Geometry: see drawing. Coordinates: mm, zero at the bounding-box minimum. Coordinates: 2 decimals unless noted, no trailing zeros. Order: outer loops, then holes, each group sorted by start corner. A loop starts at its lowest first (then second) coordinate and runs counter-clockwise, first axis right, second up. Notation, with made-up numbers: (-12.5, 81) -> (13.5, 81) arc R20 cw to (13.5, 110) -> close; hole circle Ø7 at (4, 47). An arc over 180 degrees is marked (long way). Write each question's results on one line, items separated by ' | '. Start each with the question number.
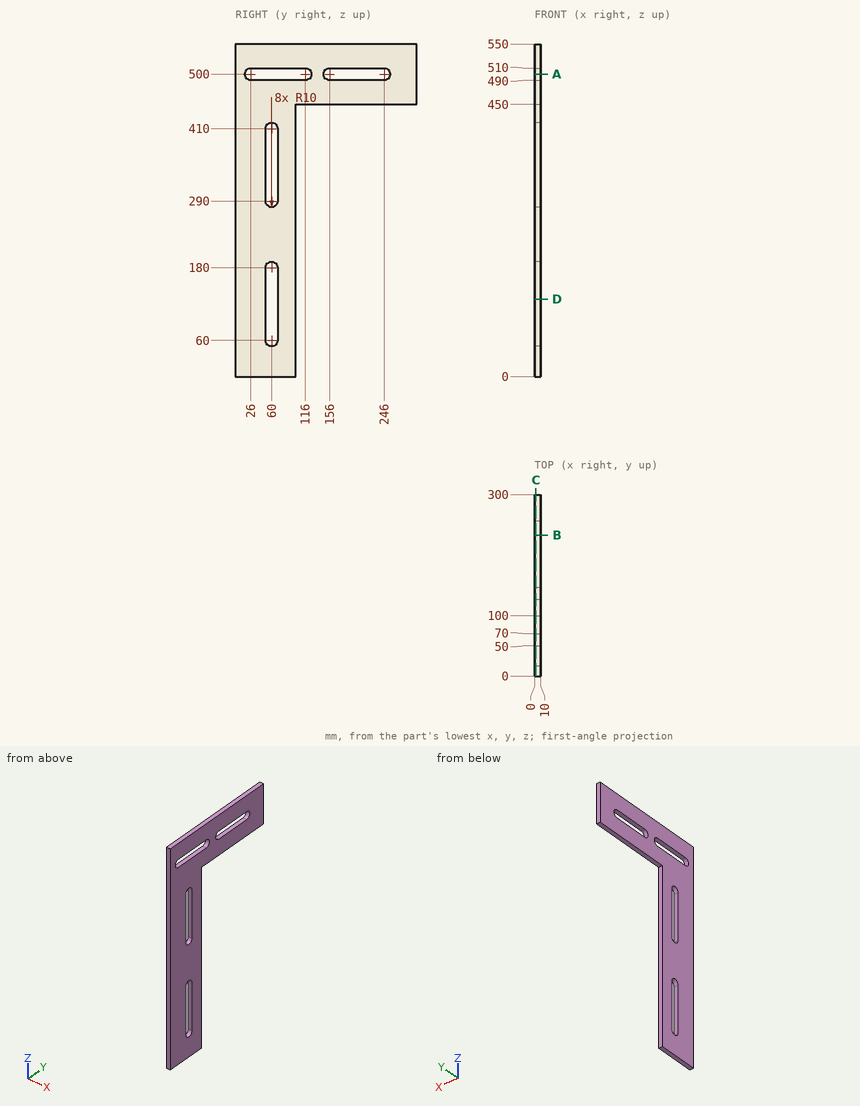
(1) Section D-D on z = 128. Return the cut outline in (x, y), then the cut area to 3 significant figures.
(2) Section B-B on y = 233. Return the cut outline in (x, z).
(3) Line query: L1, parallel to Y at x = 4.75, z = 500; L2, parallel to Y at x = 3.25, z = 403.5; L3, parallel to Z at x = 0.5, y = 180. Output: solid intervals per line, ascending.
(4) Section C-C on x = 2. Return the cut outline in (y, z), then the cut area to 3 significant figures.
(5) Section A-A on z = 500. Return the cut outline in (x, y), then the cut area to 3 significant figures.
(6) First-contact query: P1, Ø3, axis at x = 3.5, y = 187.5, coming from the -Z side; P2, Ø3, axis at x = 6, z = 329, coming from the +Y side. Flat tips, straight axial feed; report the tip coordinate or a pass-through.
Results list:
1) outline: (0, 0) -> (10, 0) -> (10, 50) -> (0, 50) -> close; (0, 70) -> (10, 70) -> (10, 100) -> (0, 100) -> close | area: 800 mm²
2) outline: (0, 450) -> (10, 450) -> (10, 490) -> (0, 490) -> close; (0, 510) -> (10, 510) -> (10, 550) -> (0, 550) -> close
3) L1: y = 0 to 16, 126 to 146, 256 to 300 | L2: y = 0 to 50, 70 to 100 | L3: z = 450 to 490, 510 to 550
4) outline: (0, 0) -> (100, 0) -> (100, 450) -> (300, 450) -> (300, 550) -> (0, 550) -> close; hole (26, 490) -> (116, 490) arc R10 ccw to (116, 510) -> (26, 510) arc R10 ccw to start; hole (50, 60) arc R10 ccw to (70, 60) -> (70, 180) arc R10 ccw to (50, 180) -> close; hole (50, 290) arc R10 ccw to (70, 290) -> (70, 410) arc R10 ccw to (50, 410) -> close; hole (156, 490) -> (246, 490) arc R10 ccw to (246, 510) -> (156, 510) arc R10 ccw to start | area: 65,300 mm²
5) outline: (0, 0) -> (10, 0) -> (10, 16) -> (0, 16) -> close; (0, 126) -> (10, 126) -> (10, 146) -> (0, 146) -> close; (0, 256) -> (10, 256) -> (10, 300) -> (0, 300) -> close | area: 800 mm²
6) P1: stops at z = 450 | P2: stops at y = 100
